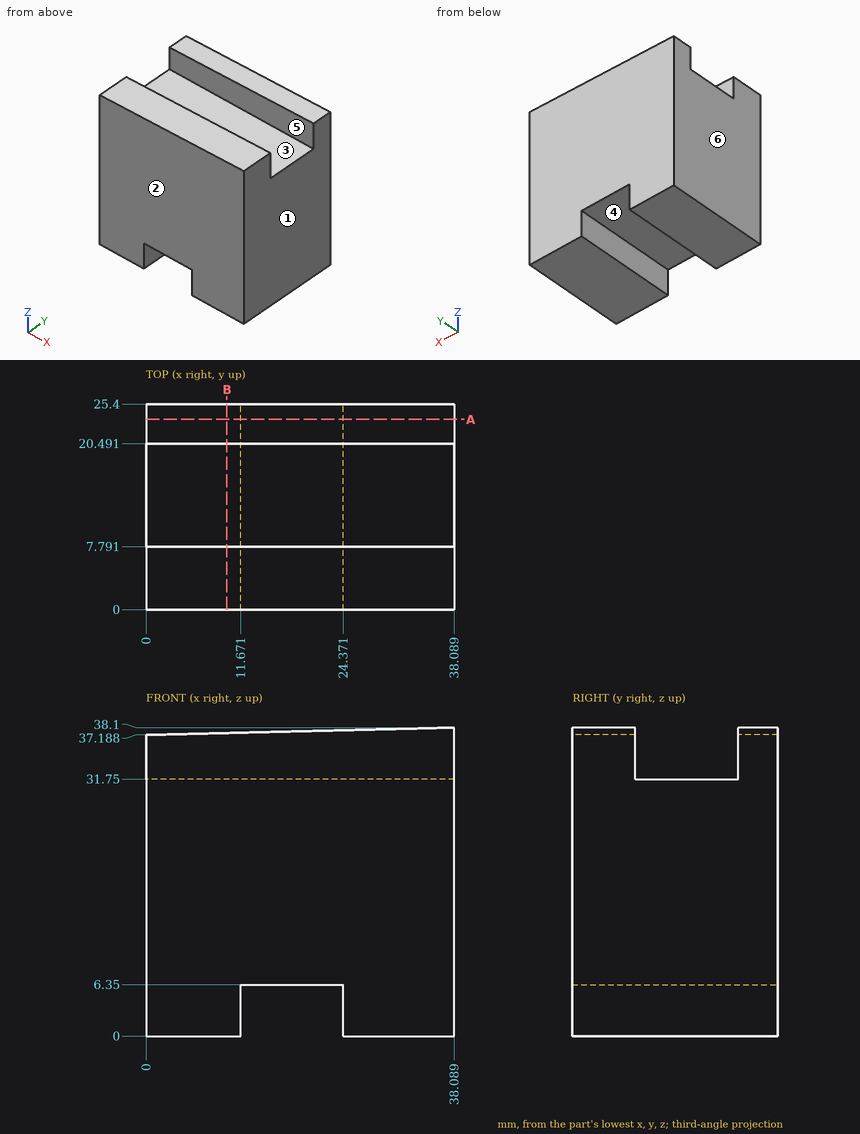
The figure shows three views and two pictorial views of one solid part (mm, origin at its lowest corner). Answer the questions. A direction names the side the tool comes from. Give positions to 0.01 mm unless a question says otherwise; leave off trailing zeros. Write each loop counter-clockwise with the first axis right and the second up, starting at its lowest first coordinate (ties: lowest second). Pieces come first, ordered by that corner, then holes. Notation, with made-up numbers: (-36, 8) -> (-10, 8) arc R5 cw to (-10, 12) -> close; hole circle Ø5 at (55, -16). An arc over 180 degrees is marked (long way). Answer as a JSON object with one key per item and string values.
1) For a pull along Y with two mould halves and no side action, classify the marked faces 1, 2 and 3 as pulls with the +Y half, pulls with the -Y half, needs draft (parallel to the pull), parting line crosses it, or undercut.
Findings below:
{"face 1": "needs draft", "face 2": "pulls with the -Y half", "face 3": "undercut"}
2) Section B-B on x = 10 is taken. Write down the section's boundary in (y, z).
Findings below:
{"outline": "(0, 0) -> (25.4, 0) -> (25.4, 37.43) -> (20.49, 37.43) -> (20.49, 31.75) -> (7.79, 31.75) -> (7.79, 37.43) -> (0, 37.43) -> close"}
3) A tool of negligible diameter and unlimited length cuts with its end or side. For the marked faces 4, 5 and 6, from which of +Z, -Z, +X, -X, +Y, -Y can it reach the whole face along a straight path? Write none if from no direction.
Findings below:
{"face 4": "-Z, +Y, -Y", "face 5": "+Z, +X, -X", "face 6": "+Z, -Z, -X, +Y, -Y"}
4) Section A-A on y = 23.5 is taken. Write down the section's boundary in (x, z).
Findings below:
{"outline": "(0, 0) -> (11.67, 0) -> (11.67, 6.35) -> (24.37, 6.35) -> (24.37, 0) -> (38.09, 0) -> (38.09, 38.1) -> (0, 37.19) -> close"}
5) Straight lines are drawn through the part: probe 1 along Y at (x, z) = (31, 33); probe 2 along Z at (x, y) = (20.5, 16.5); probe 3 along X at (y, z) = (4, 4.5). For each, find the intervals that lie inside material, in ascending order. Write a range as from..to.
Findings below:
{"probe 1": "y = 0..7.79, 20.49..25.4", "probe 2": "z = 6.35..31.75", "probe 3": "x = 0..11.67, 24.37..38.09"}
6) Flat-ended cylindrical pins translate along their axes: pin 1 Ø4 at (x, y) = (12.5, 14) entering from +Z; pin 2 Ø10 at (x, y) = (7.5, 10) entering from +Z (1 decimal); pin 3 Ø4 at (x, y) = (30, 20.5) entering from +Z. Find the tip coordinate at first contact, or state that the pin passes through.
Findings below:
{"pin 1": "stops at z = 31.75", "pin 2": "stops at z = 37.5", "pin 3": "stops at z = 37.95"}
